Geometry: final body of the model. Coordinates: model frame, mm. A direction names the side the tool comes from. Coordinates: 2 decimals unless noted, no trailing zeros. Order: outer loops, then holes, each group sorted by start corner. A loop starts at its lowest first (then second) coordinate and runs counter-clockwise, first axis right, second up. Notation, with made-up numbers: M -5,50 L 38,50 A28 cw 38,73 Z; hole C 63,-28.75 d3. An arc over 180 degrees is marked long. One line per question, with ' | ' between items.
from build123d import *

# Parameters (mm, degrees)
F0_W      = 152.4
F0_H      = 76.2
F1_DEPTH  = 50.8
F2_W      = 25.4
F2_H      = 76.2
F3_DEPTH  = 12.7
F4_W      = 25.4
F4_H      = 76.2
F5_DEPTH  = 12.7
F7_DEPTH  = 76.201
F9_DEPTH  = 76.201
F12_DEPTH = 76.201


with BuildPart() as f1:
    # F0 (on Top) → F1 (new body)
    with BuildSketch(Plane.XY):
        Rectangle(F0_W, F0_H)
    extrude(amount=F1_DEPTH)

    # F2 (on face) → F3 (cut)
    with BuildSketch(Plane.XY.offset(50.8)):
        with Locations((63.5, 0)):
            Rectangle(F2_W, F2_H)
    extrude(amount=-F3_DEPTH, mode=Mode.SUBTRACT)

    # F4 (on face) → F5 (cut)
    with BuildSketch(Plane.XY.offset(50.8)):
        with Locations((-63.5, 0)):
            Rectangle(F4_W, F4_H)
    extrude(amount=-F5_DEPTH, mode=Mode.SUBTRACT)

    # F6 (on face) → F7 (cut, through all)
    with BuildSketch(Plane.XZ.offset(38.1)):
        Polygon((-50.8, 50.8), (-50.8, 38.1), (-38.1, 38.1), align=None)
    extrude(amount=-F7_DEPTH, mode=Mode.SUBTRACT)

    # F8 (on face) → F9 (cut, through all)
    with BuildSketch(Plane.XZ.offset(38.1)):
        Polygon((38.1, 38.1), (50.8, 38.1), (50.8, 50.8), align=None)
    extrude(amount=-F9_DEPTH, mode=Mode.SUBTRACT)

    # F11 (on face) → F12 (cut, through all)
    with BuildSketch(Plane.XZ.offset(38.1)):
        Polygon((-50.802752, 12.51767), (-38.731508, 0), (38.622994, 0), (50.940588, 12.51767), align=None)
    extrude(amount=-F12_DEPTH, mode=Mode.SUBTRACT)


solid = f1.part
1. Material intervals for line 1 (Z direction, x = 47, y = 0); line 2 (Z direction, x = 43.5, y = 12); line 3 (X direction, y = 19, z = 5), sorted ascending. Write a range as [from, to].
Response values:
line 1: z = [0, 8.51], [12.52, 38.1], [47, 50.8] | line 2: z = [0, 4.96], [12.52, 38.1], [43.5, 50.8] | line 3: x = [-76.2, -43.55], [43.54, 76.2]
2. Section B-B, the plane z = 3. Output: boundary loops of the cut face in (x, y), and give its area (3 significant figures).
Response values:
outline: M -76.2,-38.1 L -41.62,-38.1 L -41.62,38.1 L -76.2,38.1 Z; M 41.58,-38.1 L 76.2,-38.1 L 76.2,38.1 L 41.58,38.1 Z | area: 5,270 mm^2
3. Section C-C, the plane x = 56. Output: boundary loops of the cut face in (y, z), and give its area (3 significant figures).
Response values:
outline: M -38.1,0 L 38.1,0 L 38.1,38.1 L -38.1,38.1 Z | area: 2,900 mm^2
4. Access query for faces 5 (the face through (-1, -38.1, 25)), 6 (the face through (-44, -1, 44)), 7 (the face through (-44.852, -0.533, 6.346)). Directions: +Z, -Z, +X, -X, +Y, -Y. A direction counts if a zero-diameter tool reaches every point of the face in a straight line with its end or side. Return the directions, or none.
Response values:
face 5: +Z, -Z, +X, -X, -Y | face 6: -X, +Y, -Y | face 7: +Y, -Y
5. Draft query along Z for faces 1 (the face through (-76.2, -1, 19)), 2 (the face through (57, 1, 38.1)), 3 (the face through (57, 1, 0)), 4 (the face through (45, -1, 45)). Return one class per face: pulls with the +Z half, pulls with the -Z half, needs draft (parallel to the pull), parting line crosses it, or undercut.
Response values:
face 1: needs draft | face 2: undercut | face 3: pulls with the -Z half | face 4: undercut
6. Pin query (flat end, axial travel): P1, Ø4, axis at y = 10.5, z = 40.5, coming from the +X side; P2, Ø10, axis at x = -7, y = -4.5, coming from the -Z side; P3, Ø19, axis at x = 62.5, y = -19, coming from the +Z side. Return the tip coordinate at first contact, or that it passes through.
Response values:
P1: stops at x = 42.5 | P2: stops at z = 12.52 | P3: stops at z = 38.1
7. Section A-A, the plane y = 13. Output: boundary loops of the cut face in (x, z).
Response values:
outline: M -76.2,0 L -38.73,0 L -50.8,12.52 L 50.94,12.52 L 38.62,0 L 76.2,0 L 76.2,38.1 L 38.1,38.1 L 50.8,50.8 L -50.8,50.8 L -38.1,38.1 L -76.2,38.1 Z
8. Section D-D, the plane z = 46. Output: boundary loops of the cut face in (x, y), and give its area (3 significant figures).
Response values:
outline: M -46,-38.1 L 46,-38.1 L 46,38.1 L -46,38.1 Z | area: 7,010 mm^2
